Can you work these out from the model? Positions are in its coordinate system, mm. Face numbers are marked on the shaded views. A direction names the side the tool comes from. Give positions to 0.01 mm unless a question says otherwise; leave off trailing zeros. Order: outer loops, then holes, each group sorted by start corner. A loop starts at its lowest first (then second) coordinate and runs counter-clockwise, first axis right, second up.
Item 1: Which directions (+Z, -Z, +X, -X, +Y, -Y) give clear straight access to the entire face, cutting with the end or side of a thin tool? Please do the marked faces 4, 5 and 6.
Item 2: I want a section at A-A, the plane z = 5. Write out the boundary of the cut face in (x, y), then the cut area to 3 significant figures.
Item 3: I'm going to push a flat-ended pin straight in: pin 1 Ø0.8 at (x, z) = (5, 6.5) entering from -Y. Where does the tip first touch, or does it pass through?
Item 4: I want a section at B-B, the plane x = -1.25. Write out the boundary of the cut face in (y, z).
Item 5: If I drill on line 1 along X through (y, z) = (-1.6, 5); line 2 along Z through (x, y) = (0, 1); line 3 along X through (y, z) = (-0.55, 4.5), over which ranges is the centre line in solid material (lowest first)?
Item 6: I want a section at D-D, the plane z = 1.25. Write out the boundary of the cut face in (x, y), then the cut area to 3 significant figures.
Item 7: I want a section at C-C, the plane y = -2.65. Write out the boundary of the cut face in (x, z).
Item 8: If we mould it in two halves opening along Z, with no side actions, what happens to the marked faces 1, 2 and 3? For each: +Z half, -Z half, draft (parallel to the pull), parting line (faces both ways), or undercut.
Autodesk Inventor part; units mm, degrees
ref_plane "YZ Plane" through (0, 0, 0) normal (1, 0, 0) x (0, 1, 0)
ref_plane "XZ Plane" through (0, 0, 0) normal (0, 1, 0) x (-1, 0, 0)
ref_plane "XY Plane" through (0, 0, 0) normal (0, 0, 1) x (1, 0, 0)
sketch "Skizze1" plane through (0, 0, 0) normal (0, 0, 1) x (1, 0, 0)
  line L0 (-2.7002, -2.1223) -> (-2.7002, -3.4436)
  line L1 (-5.4502, -2.1223) -> (-2.7002, -2.1223)
  line L2 (-5.4502, -1.2612) -> (-5.4502, -2.1223)
  line L3 (-2.6446, 1.5444) -> (-5.4502, -1.2612)
  line L4 (0.3248, 1.5444) -> (-2.6446, 1.5444)
  line L5 (2.7441, 1.5444) -> (0.3248, 1.5444)
  line L6 (5.5498, -1.2612) -> (2.7441, 1.5444)
  line L7 (5.5498, -2.1223) -> (5.5498, -1.2612)
  line L8 (2.7998, -2.1223) -> (5.5498, -2.1223)
  line L9 (2.7998, -3.4436) -> (2.7998, -2.1223)
  line L10 (-2.7002, -3.4436) -> (2.7998, -3.4436)
  point P0 (0, 0)
  dimension "d0" = 11
  dimension "d1" = 1.5444
extrude "Extrusion1" add sketch "Skizze1" along normal blind 10
sketch "Skizze2" plane through (-2.6446, 1.5444, 0) normal (0, 1, 0) x (1, 0, 0)
  line L0 (5.3888, 0) -> (0, 0)
  line L1 (0, 0) -> (0, -10)
  line L2 (5.3888, -10) -> (0, -10)
  line L3 (5.3888, 0) -> (5.3888, -10)
  circle A0 centre (2.6944, -5) radius 2.1
  point P0 (2.6446, 0)
  dimension "d4" = 4.2
extrude "Extrusion2" cut sketch "Skizze2" against normal up to surface (4.988 mm away) contours A0
properties part number "T-Brick"
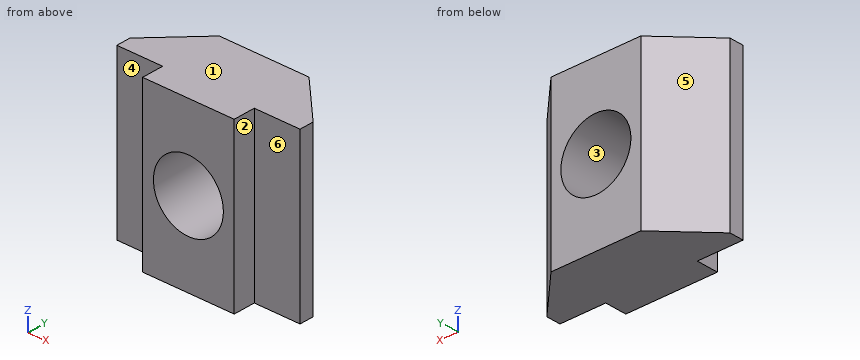
Results list:
1. face 4: +Z, -Z, -X, -Y
1. face 5: +Z, -Z, -X, +Y
1. face 6: +Z, -Z, +X, -Y
2. outline: (-5.45, -2.12) - (-2.7, -2.12) - (-2.7, -3.44) - (-2.05, -3.44) - (-2.05, 1.54) - (-2.64, 1.54) - (-5.45, -1.26) - close; (2.15, -3.44) - (2.8, -3.44) - (2.8, -2.12) - (5.55, -2.12) - (5.55, -1.26) - (2.74, 1.54) - (2.15, 1.54) - close
2. area: 18.8 mm2
3. pin 1: stops at y = -2.12
4. outline: (-3.44, 0) - (1.54, 0) - (1.54, 3.35) - (-3.44, 3.35) - close; (-3.44, 6.65) - (1.54, 6.65) - (1.54, 10) - (-3.44, 10) - close
5. line 1: x = -5.45 to -2.05, 2.15 to 5.55
5. line 2: z = 0 to 2.9, 7.1 to 10
5. line 3: x = -4.74 to -1.99, 2.09 to 4.84
6. outline: (-5.45, -2.12) - (-2.7, -2.12) - (-2.7, -3.44) - (2.8, -3.44) - (2.8, -2.12) - (5.55, -2.12) - (5.55, -1.26) - (2.74, 1.54) - (-2.64, 1.54) - (-5.45, -1.26) - close
6. area: 39.7 mm2
7. outline: (-2.7, 0) - (2.8, 0) - (2.8, 10) - (-2.7, 10) - close; hole circle Ø4.2 at (0.05, 5)
8. face 1: +Z half
8. face 2: draft
8. face 3: undercut
